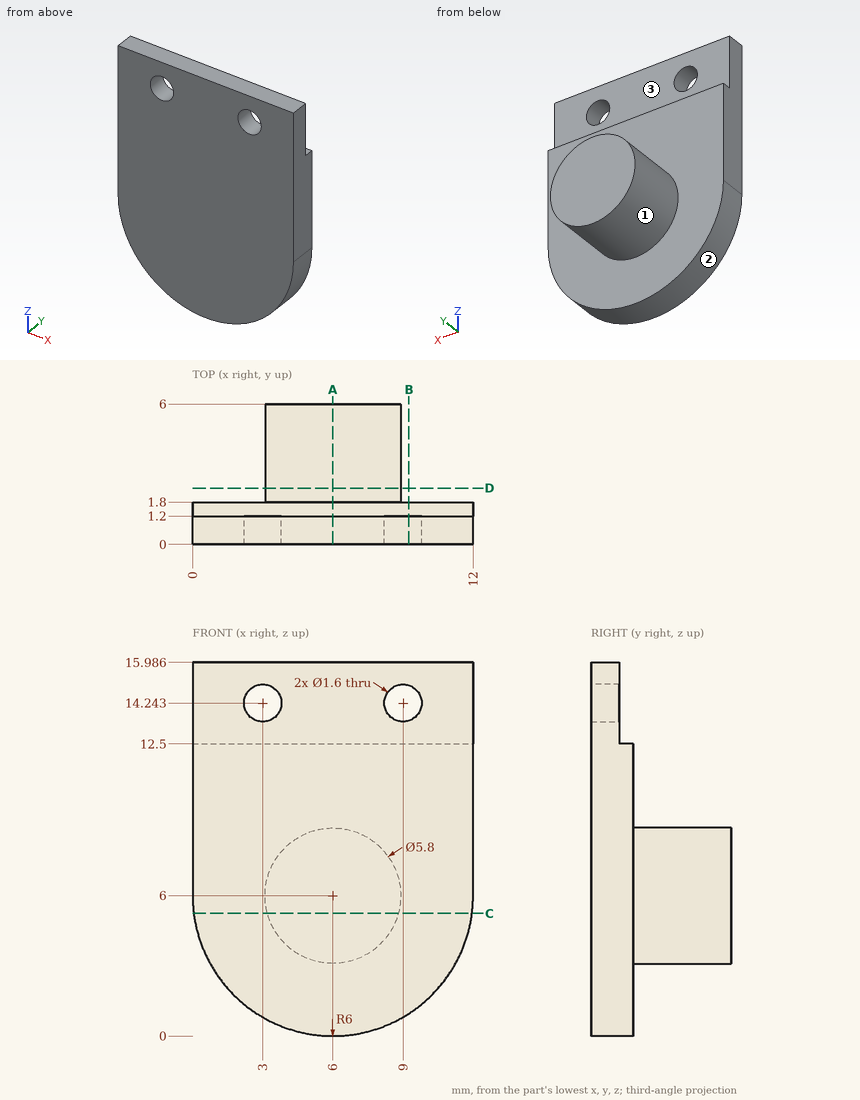
The figure shows three views and two pictorial views of one solid part (mm, origin at its lowest corner). Answer the questions. A direction names the side the tool comes from. Round coordinates to 2 decimals unless told otherwise and drop trailing zeros. Write each loop counter-clockwise with the first axis right and the second up, starting at its lowest first coordinate (ties: lowest second). Pieces come first, ordered by that corner, then holes. Notation, with made-up numbers: (15, 74.25) - (27, 74.25) arc R23 cw to (27, 113.25) - close; hole circle Ø6 at (43.5, -8). An arc over 180 degrees is marked (long way). Use one line per item in the form item = value. Start each with the question number.
Item 1: A cutting plane is placed at B-B (x = 9.25). Write down the section's boundary in (y, z).
Item 2: Find the intervals of material crossed by line 1 (Y direction, x = 2.5, z = 3); line 2 (Y direction, x = 11.75, z = 14.25); line 3 (X direction, y = 2.1, z = 6), in increasing order. Write a range as [from, to].
Item 3: A cutting plane is placed at C-C (z = 5.25). Write down the section's boundary in (x, y).
Item 4: A cutting plane is placed at A-A (x = 6). Write down the section's boundary in (y, z).
Item 5: A cutting plane is placed at D-D (y = 2.4). Write down the section's boundary in (x, z).
Item 6: Flat-ended cylindrical pins translate along their axes: pin 1 Ø1.5 at (y, z) = (3.5, 8) entering from +X; pin 2 Ø1 at (x, z) = (5.5, 13.5) entering from +Y. Find the tip coordinate at first contact, or state that the pin passes through.
Item 7: A tool of negligible diameter and unlimited length cuts with its end or side. For the marked faces 1, 2 and 3, from which of +Z, -Z, +X, -X, +Y, -Y can it reach the whole face along a straight path? Write none if from no direction.
The answers:
q1.outline = (0, 0.96) - (1.8, 0.96) - (1.8, 12.5) - (1.2, 12.5) - (1.2, 13.48) - (0, 13.48) - close; (0, 15) - (1.2, 15) - (1.2, 15.99) - (0, 15.99) - close
q2.line_1 = [0, 1.8]
q2.line_2 = [0, 1.2]
q2.line_3 = [3.1, 8.9]
q3.outline = (0.05, 0) - (11.95, 0) - (11.95, 1.8) - (8.8, 1.8) - (8.8, 6) - (3.2, 6) - (3.2, 1.8) - (0.05, 1.8) - close
q4.outline = (0, 0) - (1.8, 0) - (1.8, 3.1) - (6, 3.1) - (6, 8.9) - (1.8, 8.9) - (1.8, 12.5) - (1.2, 12.5) - (1.2, 15.99) - (0, 15.99) - close
q5.outline = circle Ø5.8 at (6, 6)
q6.pin_1 = 8.62
q6.pin_2 = 1.2
q7.face_1 = +Y
q7.face_2 = -Z, +Y, -Y
q7.face_3 = +Z, +X, -X, +Y
